from build123d import *

# Parameters (mm, degrees)
SKETCH1_W                     = 127.635
SKETCH1_H                     = 127.635
BOSS_EXTRUDE1_DEPTH           = 9.525
SKETCH5_W                     = 108.585
SKETCH5_H                     = 108.585
CUT_EXTRUDE1_DEPTH            = 9.525
FILLET1_R                     = 6.35
TAP_DRILL_FOR_6_32_TAP2_D     = 2.7051
TAP_DRILL_FOR_6_32_TAP2_DEPTH = 12.7
TAP_DRILL_FOR_6_32_TAP2_TIP   = 0.81269403
TAP_DRILL_FOR_6_32_TAP3_D     = 2.7051
TAP_DRILL_FOR_6_32_TAP3_DEPTH = 12.7
TAP_DRILL_FOR_6_32_TAP3_TIP   = 0.81269403
TAP_DRILL_FOR_6_32_TAP4_D     = 2.7051
TAP_DRILL_FOR_6_32_TAP4_DEPTH = 12.7
TAP_DRILL_FOR_6_32_TAP4_TIP   = 0.81269403
TAP_DRILL_FOR_6_32_TAP5_D     = 2.7051
TAP_DRILL_FOR_6_32_TAP5_DEPTH = 12.7
TAP_DRILL_FOR_6_32_TAP5_TIP   = 0.81269403


with BuildPart() as part:
    # Sketch1 → Boss-Extrude1 (new body)
    with BuildSketch(Plane(origin=(0, 0, 0), x_dir=(1, 0, 0), z_dir=(0, 1, 0))):
        with Locations((63.8175, 63.8175)):
            Rectangle(SKETCH1_W, SKETCH1_H)
    extrude(amount=BOSS_EXTRUDE1_DEPTH)

    # Sketch5 → Cut-Extrude1 (cut)
    with BuildSketch(Plane(origin=(0, 9.525, 0), x_dir=(1, 0, 0), z_dir=(0, 1, 0))):
        with Locations((63.8175, 63.8175)):
            Rectangle(SKETCH5_W, SKETCH5_H)
    extrude(amount=-CUT_EXTRUDE1_DEPTH, mode=Mode.SUBTRACT)

    # Fillet1
    fillet1_edges = [part.edges().sort_by_distance(p)[0] for p in [
        (118.11, 4.7625, -9.525),
        (9.525, 4.7625, -9.525),
        (9.525, 4.7625, -118.11),
        (118.11, 4.7625, -118.11),
    ]]
    fillet(fillet1_edges, radius=FILLET1_R)

    # Tap Drill for #6-32 Tap2
    with Locations(Plane(origin=(127.635, 0, 0), x_dir=(0, 0, -1), z_dir=(1, 0, 0))):
        with Locations((4.7625, 4.7625)):
            Hole(TAP_DRILL_FOR_6_32_TAP2_D / 2, depth=TAP_DRILL_FOR_6_32_TAP2_DEPTH)
            with Locations((0, 0, -(TAP_DRILL_FOR_6_32_TAP2_DEPTH + TAP_DRILL_FOR_6_32_TAP2_TIP / 2))):  # 118° drill point
                Cone(0, TAP_DRILL_FOR_6_32_TAP2_D / 2, TAP_DRILL_FOR_6_32_TAP2_TIP, mode=Mode.SUBTRACT)

    # Tap Drill for #6-32 Tap3
    with Locations(Plane.XY):
        with Locations((4.7625, 4.7625)):
            Hole(TAP_DRILL_FOR_6_32_TAP3_D / 2, depth=TAP_DRILL_FOR_6_32_TAP3_DEPTH)
            with Locations((0, 0, -(TAP_DRILL_FOR_6_32_TAP3_DEPTH + TAP_DRILL_FOR_6_32_TAP3_TIP / 2))):  # 118° drill point
                Cone(0, TAP_DRILL_FOR_6_32_TAP3_D / 2, TAP_DRILL_FOR_6_32_TAP3_TIP, mode=Mode.SUBTRACT)

    # Tap Drill for #6-32 Tap4
    with Locations(Plane.ZY):
        with Locations((-122.8725, 4.7625)):
            Hole(TAP_DRILL_FOR_6_32_TAP4_D / 2, depth=TAP_DRILL_FOR_6_32_TAP4_DEPTH)
            with Locations((0, 0, -(TAP_DRILL_FOR_6_32_TAP4_DEPTH + TAP_DRILL_FOR_6_32_TAP4_TIP / 2))):  # 118° drill point
                Cone(0, TAP_DRILL_FOR_6_32_TAP4_D / 2, TAP_DRILL_FOR_6_32_TAP4_TIP, mode=Mode.SUBTRACT)

    # Tap Drill for #6-32 Tap5
    with Locations(Plane(origin=(0, 0, -127.635), x_dir=(-1, 0, 0), z_dir=(0, 0, -1))):
        with Locations((-122.8725, 4.7625)):
            Hole(TAP_DRILL_FOR_6_32_TAP5_D / 2, depth=TAP_DRILL_FOR_6_32_TAP5_DEPTH)
            with Locations((0, 0, -(TAP_DRILL_FOR_6_32_TAP5_DEPTH + TAP_DRILL_FOR_6_32_TAP5_TIP / 2))):  # 118° drill point
                Cone(0, TAP_DRILL_FOR_6_32_TAP5_D / 2, TAP_DRILL_FOR_6_32_TAP5_TIP, mode=Mode.SUBTRACT)


solid = part.part
Geometry check sheet. Reference: the model listing, model coordinates, mm. A direction names the side the tool comes from. Coordinates: 2 decimals unless noted, no trailing zeros. Order: outer loops, then holes, each group sorted by start corner. A loop starts at its lowest first (then second) coordinate and runs counter-clockwise, first axis right, second up. Notation, with made-up numbers: (42.5, 15.25) - (50.5, 15.25) arc R7 cw to (50.5, 23.25) - close; hole circle Ø3 at (76, 80). An arc over 180 degrees is marked (long way). One line per item, written item: value.
(1) Thickness scan on probe 1 along Z at (x, y) = (45.5, 3.25) (3 decimals); probe 2 along X at (y, z) = (4.5, -45.5) (3 decimals); probe 3 along Z at (x, y) = (15, 2) (3 decimals). Record the ranges inside material, lowest first. Write a range as from..to.
Data:
probe 1: z = -127.635..-118.11, -9.525..0
probe 2: x = 0..9.525, 118.11..127.635
probe 3: z = -127.635..-118.049, -9.586..0
(2) Sectioned sample at B-B (x = 70). Enter the section's corners in (y, z) (3 decimals), and give its area (3 significant figures).
Data:
outline: (0, -127.635) - (9.525, -127.635) - (9.525, -118.11) - (0, -118.11) - close; (0, -9.525) - (9.525, -9.525) - (9.525, 0) - (0, 0) - close
area: 181 mm^2
(3) Sectioned sample at A-A (z = -55). Enter the section's corners in (x, y) (3 decimals), and give its area (3 significant figures).
Data:
outline: (0, 0) - (9.525, 0) - (9.525, 9.525) - (0, 9.525) - close; (118.11, 0) - (127.635, 0) - (127.635, 9.525) - (118.11, 9.525) - close
area: 181 mm^2
(4) Depth check by flat-ended pin: pin 1 Ø2 at (y, z) = (4.76, -4.76) entering from +X. Enter the tip coordinate at first touch or a pass-through.
Data:
pin 1: stops at x = 114.73
(5) Release check for a two-part mould opening along X. For faces 1 (the face through (127.635, 5, -63)), 2 (the face through (63, 5, -127.635)), 3 (the face through (63, 5, -118.11)), 4 (the face through (0, 5, -63)) record: +X half, -X half, draft (parallel to the pull), parting line (faces both ways), or undercut.
Data:
face 1: +X half
face 2: draft
face 3: undercut
face 4: -X half
(6) Access from +Z, -Z, +X, -X, +Y, -Y to the whole of each face (thin tool, end or side, straight path). Record for faces 5 (the face through (116.2, 4.696, -11.336)), 6 (the face through (63, 5, 0)).
Data:
face 5: +Y, -Y
face 6: +Z, +X, -X, +Y, -Y
